Geometry check sheet. Reference: the model listing, model coordinates, mm. A direction names the side the tool comes from. Round coordinates to 2 decimals unless told otherwise and drop trailing zeros. Order: outer loops, then holes, each group sorted by start corner. A loop starts at its lowest first (then second) coordinate and runs counter-clockwise, first axis right, second up. Notation, with made-up numbers: M 8,2.5 L 35,2.5 A23 ccw 35,15.5 Z; hole C 52,-30.5 d5. An arc over 180 degrees is marked long. Return JSON: item names as keys, results as strings. Group by question number.
```python
from build123d import *

# Parameters (mm, degrees)
SKETCH_2_W          = 129.667
SKETCH_2_H          = 78.613
EXTRUDE_1_DEPTH     = 0.8
SKETCH_3_R          = 1.27
CUT_EXTRUDE_1_DEPTH = 12.54
SKETCH_4_R          = 0.92202
SKETCH_4_R_2        = 0.922029104
SKETCH_4_R_3        = 0.919681264
SKETCH_4_R_4        = 0.924963229
SKETCH_4_R_5        = 0.92552898
EXTRUDE_2_DEPTH     = 1
SKETCH_5_W          = 38
SKETCH_5_H          = 12
EXTRUDE_3_DEPTH     = 2.2
SKETCH_6_W          = 30
SKETCH_6_H          = 12
EXTRUDE_4_DEPTH     = 1.2


with BuildPart() as part:
    # 草图2 → 凸台-拉伸1 (new body)
    with BuildSketch(Plane.XY):
        with Locations((83.3755, 41.2115)):
            Rectangle(SKETCH_2_W, SKETCH_2_H)
    extrude(amount=EXTRUDE_1_DEPTH)

    # 草图3 → 切除-拉伸1 (cut)
    with BuildSketch(Plane.XY.offset(0.8)):
        with Locations((33.02, 77.978)):
            Circle(SKETCH_3_R)
        with Locations((81.28, 78.105)):
            Circle(SKETCH_3_R)
        with Locations((127, 77.978)):
            Circle(SKETCH_3_R)
        with Locations((33.02, 4.953)):
            Circle(SKETCH_3_R)
        with Locations((81.28, 4.953)):
            Circle(SKETCH_3_R)
        with Locations((127.127, 5.08)):
            Circle(SKETCH_3_R)
    extrude(amount=-CUT_EXTRUDE_1_DEPTH, mode=Mode.SUBTRACT)

    # 草图4 → 凸台-拉伸2 (add)
    with BuildSketch(Plane.XY.offset(0.8)):
        with Locations((22.098, 72.009)):
            Circle(SKETCH_4_R)
        with Locations((22.098, 64.643)):
            Circle(SKETCH_4_R)
        with Locations((22.098, 56.769)):
            Circle(SKETCH_4_R)
        with Locations((22.098, 49.149)):
            Circle(SKETCH_4_R)
        with Locations((22.098, 26.162)):
            Circle(SKETCH_4_R)
        with Locations((22.098, 33.528)):
            Circle(SKETCH_4_R)
        with Locations((22.098, 41.275)):
            Circle(SKETCH_4_R)
        with Locations((32.258, 72.009)):
            Circle(SKETCH_4_R)
        with Locations((42.926, 71.882)):
            Circle(SKETCH_4_R)
        with Locations((53.086, 72.009)):
            Circle(SKETCH_4_R)
        with Locations((63.246, 71.882)):
            Circle(SKETCH_4_R)
        with Locations((73.533, 71.882)):
            Circle(SKETCH_4_R)
        with Locations((83.693, 71.882)):
            Circle(SKETCH_4_R)
        with Locations((94.361, 71.882)):
            Circle(SKETCH_4_R)
        with Locations((104.648, 71.882)):
            Circle(SKETCH_4_R)
        with Locations((114.808, 71.882)):
            Circle(SKETCH_4_R)
        with Locations((124.968, 71.882)):
            Circle(SKETCH_4_R)
        with Locations((135.255, 71.882)):
            Circle(SKETCH_4_R)
        with Locations((32.385, 64.516)):
            Circle(SKETCH_4_R)
        with Locations((32.385, 56.769)):
            Circle(SKETCH_4_R)
        with Locations((32.258, 49.022)):
            Circle(SKETCH_4_R)
        with Locations((32.258, 33.528)):
            Circle(SKETCH_4_R)
        with Locations((32.258, 41.275)):
            Circle(SKETCH_4_R)
        with Locations((54.102, 26.162)):
            Circle(SKETCH_4_R)
        with Locations((30.099, 26.162)):
            Circle(SKETCH_4_R)
        with Locations((38.1, 26.162)):
            Circle(SKETCH_4_R)
        with Locations((46.101, 26.162)):
            Circle(SKETCH_4_R)
        with Locations((42.926, 64.643)):
            Circle(SKETCH_4_R)
        with Locations((42.799, 56.769)):
            Circle(SKETCH_4_R)
        with Locations((53.086, 64.516)):
            Circle(SKETCH_4_R)
        with Locations((63.246, 64.516)):
            Circle(SKETCH_4_R)
        with Locations((53.086, 56.769)):
            Circle(SKETCH_4_R)
        with Locations((63.246, 56.769)):
            Circle(SKETCH_4_R)
        with Locations((42.937232377, 49.080669284)):
            Circle(SKETCH_4_R)
        with Locations((53.086, 49.022)):
            Circle(SKETCH_4_R)
        with Locations((63.246, 49.022)):
            Circle(SKETCH_4_R)
        with Locations((42.927878215, 41.278345649)):
            Circle(SKETCH_4_R)
        with Locations((42.78999374, 33.521368778)):
            Circle(SKETCH_4_R)
        with Locations((53.086, 33.528)):
            Circle(SKETCH_4_R)
        with Locations((53.096022403, 41.290450758)):
            Circle(SKETCH_4_R)
        with Locations((104.775, 4.699)):
            Circle(SKETCH_4_R)
        with Locations((116.84, 9.652)):
            Circle(SKETCH_4_R_2)
        with Locations((109.855, 16.891)):
            Circle(SKETCH_4_R)
        with Locations((124.333, 16.764)):
            Circle(SKETCH_4_R_3)
        with Locations((116.84, 24.257)):
            Circle(SKETCH_4_R_4)
        with Locations((135.255, 33.528)):
            Circle(SKETCH_4_R_5)
        with Locations((135.255, 41.275)):
            Circle(SKETCH_4_R)
        with Locations((124.968, 33.401)):
            Circle(SKETCH_4_R)
        with Locations((124.968, 41.275)):
            Circle(SKETCH_4_R)
        with Locations((114.808, 33.401)):
            Circle(SKETCH_4_R)
        with Locations((114.808, 41.148)):
            Circle(SKETCH_4_R)
        with Locations((130.175, 48.895)):
            Circle(SKETCH_4_R)
        with Locations((122.174, 48.895)):
            Circle(SKETCH_4_R)
        with Locations((114.808, 48.895)):
            Circle(SKETCH_4_R)
        with Locations((124.968, 56.769)):
            Circle(SKETCH_4_R)
        with Locations((114.808, 56.769)):
            Circle(SKETCH_4_R)
        with Locations((114.808, 64.516)):
            Circle(SKETCH_4_R)
        with Locations((124.968, 64.516)):
            Circle(SKETCH_4_R)
        with Locations((135.255, 64.516)):
            Circle(SKETCH_4_R)
        with Locations((62.103, 26.162)):
            Circle(SKETCH_4_R)
        with Locations((70.104, 26.162)):
            Circle(SKETCH_4_R)
        with Locations((63.373, 33.528)):
            Circle(SKETCH_4_R)
        with Locations((78.74, 33.528)):
            Circle(SKETCH_4_R)
        with Locations((87.122, 33.528)):
            Circle(SKETCH_4_R)
        with Locations((104.521, 33.528)):
            Circle(SKETCH_4_R)
        with Locations((94.361, 33.401)):
            Circle(SKETCH_4_R)
        with Locations((73.533, 41.275)):
            Circle(SKETCH_4_R)
        with Locations((63.246, 41.275)):
            Circle(SKETCH_4_R)
        with Locations((83.693, 41.275)):
            Circle(SKETCH_4_R)
        with Locations((104.648, 41.275)):
            Circle(SKETCH_4_R)
        with Locations((94.361, 41.148)):
            Circle(SKETCH_4_R)
        with Locations((73.533, 49.022)):
            Circle(SKETCH_4_R)
        with Locations((83.693, 49.022)):
            Circle(SKETCH_4_R)
        with Locations((94.361, 49.022)):
            Circle(SKETCH_4_R)
        with Locations((104.521, 49.022)):
            Circle(SKETCH_4_R)
        with Locations((73.533, 64.516)):
            Circle(SKETCH_4_R)
        with Locations((73.533, 56.769)):
            Circle(SKETCH_4_R)
        with Locations((83.693, 64.516)):
            Circle(SKETCH_4_R)
        with Locations((83.693, 56.769)):
            Circle(SKETCH_4_R)
        with Locations((94.361, 64.516)):
            Circle(SKETCH_4_R)
        with Locations((94.361, 56.642)):
            Circle(SKETCH_4_R)
        with Locations((104.521, 56.642)):
            Circle(SKETCH_4_R)
        with Locations((104.648, 64.516)):
            Circle(SKETCH_4_R)
        with Locations((135.255, 56.642)):
            Circle(SKETCH_4_R)
    extrude(amount=EXTRUDE_2_DEPTH)

    # 草图5 → 凸台-拉伸3 (add)
    with BuildSketch(Plane.XY.offset(0.8)):
        with Locations((46.17406, 13.42438)):
            Rectangle(SKETCH_5_W, SKETCH_5_H)
    extrude(amount=EXTRUDE_3_DEPTH)

    # 草图6 → 凸台-拉伸4 (add)
    with BuildSketch(Plane.XY.offset(3)):
        with Locations((47.17406, 13.42438)):
            Rectangle(SKETCH_6_W, SKETCH_6_H)
    extrude(amount=EXTRUDE_4_DEPTH)


solid = part.part
```
Q1. Set-up check for faces 4 (the face through (46, 19.424, 2)), 5 (the face through (30, 14, 3)), 6 (the face through (80.01, 5.01, 0.41)), 7 (the face through (82, 42, 0.8)): record each of +Z, -Z, +X, -X, +Y, -Y from which the full face is reachable in a straight line by a thin tool's end or side.
Q2. Section check A-A on x = 49.5. Record the cut outline in (y, z) (3 decimals).
Q3. Release check for a two-part mould opening along Y. For faces 1 (the face through (46, 7.424, 2)), 2 (the face through (64, 14, 3)), 3 (the face through (80.3, 77.3, 0.4)) record: +Y half, -Y half, draft (parallel to the pull), parting line (faces both ways), or undercut.
Q4. Material ranges on line 1 along Y through (x, z) = (81.28, 0.65) (3 decimals); line 2 along Y through (x, z) = (33.02, 0.3) (3 decimals); line 3 along Z through (x, y) = (91, 27), recorded low to high.
Q5. Section check B-B on y = 21. Record the cut outline in (x, z).
Q6. Depth check by flat-ended pin: pin 1 Ø2 at (x, y) = (33, 61) entering from +Z; pin 2 Ø0.9 at (x, y) = (104.5, 5) entering from +Z; pin 3 Ø2 at (y, z) = (49, 3.5) entering from -X; pin 4 Ø6 at (x, y) = (72, 48) entering from -Z. Enter the tip coordinate at first touch or a pass-through.
Geometry check:
{
 "1": {"face 4": "+Z, +X, -X", "face 5": "+Z, -X, +Y, -Y", "face 6": "+Z, -Z", "face 7": "+Z"},
 "2": {"outline": "M 1.905,0 L 80.518,0 L 80.518,0.8 L 19.424,0.8 L 19.424,4.2 L 7.424,4.2 L 7.424,0.8 L 1.905,0.8 Z"},
 "3": {"face 1": "-Y half", "face 2": "draft", "face 3": "undercut"},
 "4": {"line 1": "y = 1.905 to 3.683, 6.223 to 76.835, 79.375 to 80.518", "line 2": "y = 1.905 to 3.683, 6.223 to 76.708, 79.248 to 80.518", "line 3": "z = 0 to 0.8"},
 "5": {"outline": "M 18.54,0 L 148.21,0 L 148.21,0.8 L 18.54,0.8 Z"},
 "6": {"pin 1": "stops at z = 0.8", "pin 2": "stops at z = 1.8", "pin 3": "passes through", "pin 4": "stops at z = 0"}
}
